Here's the drawing with two shaded views (mm, measured from the low corner). I have some questions. A direction names the side the tool comes from. Round coordinates to 2 decimals unless told otherwise and drop trailing zeros. Loops run counter-clockwise (first coordinate to the right, second up) from the corner with the lowest first, then second, coordinate; pieces in that order, holes last. Notation, with made-up numbers: (49, 17.5) -> (78, 17.5) arc R21 ccw to (78, 38.5) -> close; hole circle Ø1 at (-22.75, 56.25). An arc over 180 degrees is marked (long way). Write each question's results on one line, items separated by ' | '. Start each with the question number.
1) For P1, Ø3, axis at y = 4, z = 0.5, coming from the -X side; P2, Ø2, axis at x = 4, y = 2.5, coming from the -Z side, each with a flat end and sliding along its axis, tell me the tip position at first contact or that it passes through.
2) Imagine slicing it at C-C, the plane y = 0.75. List the corners of the cut face in (x, z) for me, plus the area to 3 significant figures.
3) Which directions (+Z, -Z, +X, -X, +Y, -Y) give clear straight access to the entire face, cutting with the end or side of a thin tool? Please do the marked faces 1 and 2.
4) Imagine slicing it at D-D, the plane y = 4.25. List the corners of the cut face in (x, z) for me.
5) If I drill on probe 1 along Y at (x, z) = (1.3, 0.5); probe 2 along Z at (x, y) = (0.5, 1.75); probe 3 along Z at (x, y) = (3.85, 2), over which ranges is the centre line in solid material (lowest first)?
6) Imagine slicing it at A-A, the plane x = 2.5. List the corners of the cut face in (y, z) for me, plus the area to 3 significant figures.
7) Imagine slicing it at B-B, the plane z = 2.5. List the corners of the cut face in (x, y) for me, plus the area to 3 significant figures.
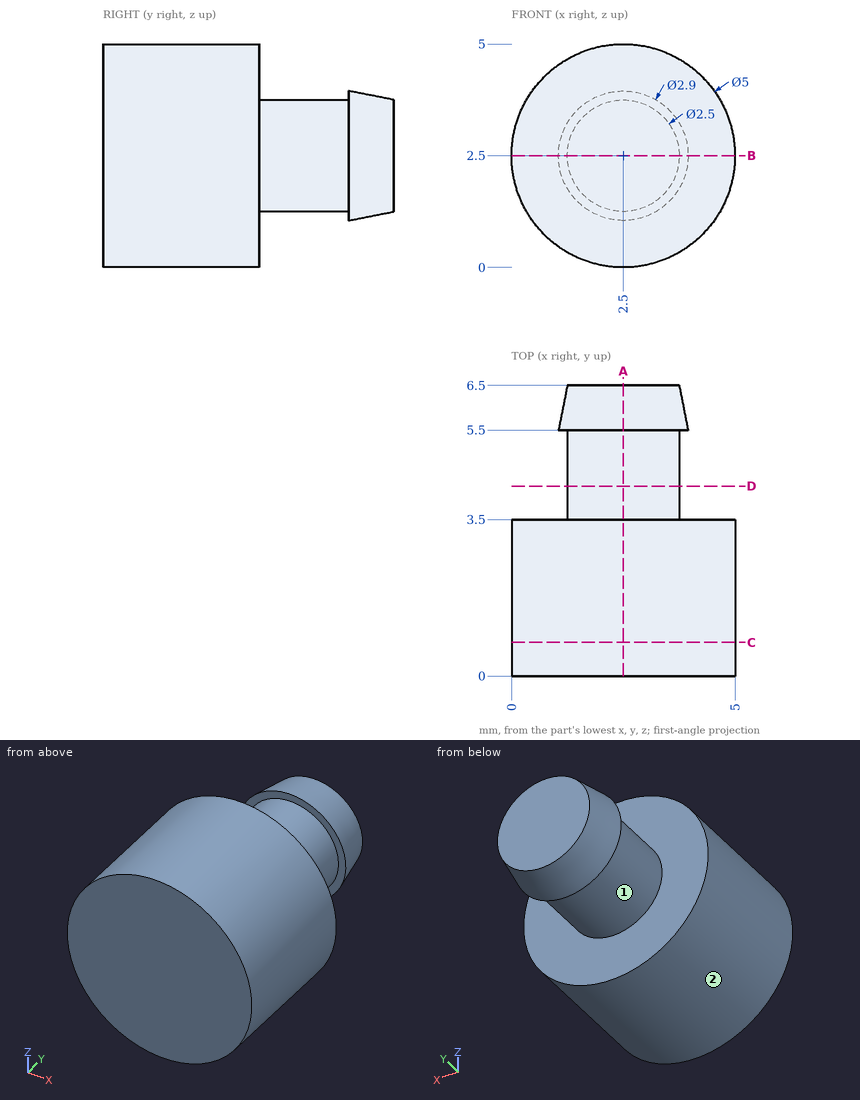
Checked values:
1) P1: x = 0.07 | P2: z = 0.05
2) outline: circle Ø5 at (2.5, 2.5) | area: 19.6 mm^2
3) face 1: none | face 2: +Y, -Y
4) outline: circle Ø2.5 at (2.5, 2.5)
5) probe 1: 0 to 3.5 | probe 2: 1 to 4 | probe 3: 0.4 to 4.6
6) outline: (0, 0) -> (3.5, 0) -> (3.5, 1.25) -> (5.5, 1.25) -> (5.5, 1.05) -> (6.5, 1.25) -> (6.5, 3.75) -> (5.5, 3.95) -> (5.5, 3.75) -> (3.5, 3.75) -> (3.5, 5) -> (0, 5) -> close | area: 25.2 mm^2
7) outline: (0, 0) -> (5, 0) -> (5, 3.5) -> (3.75, 3.5) -> (3.75, 5.5) -> (3.95, 5.5) -> (3.75, 6.5) -> (1.25, 6.5) -> (1.05, 5.5) -> (1.25, 5.5) -> (1.25, 3.5) -> (0, 3.5) -> close | area: 25.2 mm^2
